```python
from build123d import *

# Parameters (mm, degrees)
SALIENTE_EXTRUIR4_DEPTH = 20
SALIENTE_EXTRUIR5_DEPTH = 30


with BuildPart() as part:
    # Croquis2 → Saliente-Extruir4 (new body)
    with BuildSketch(Plane(origin=(0, 0, 0), x_dir=(1, 0, 0), z_dir=(0, 1, 0))):
        Polygon((130, 20.207259422), (130, 24.997259422), (60, 24.997259422), (60, 44.997259422), (130, 44.997259422), (130, 49.792740578), (95, 70), (0, 70), (0, 0), (95, 0), align=None)
    extrude(amount=SALIENTE_EXTRUIR4_DEPTH)

    # Croquis4 → Saliente-Extruir5 (add)
    with BuildSketch(Plane.ZY):
        Polygon((0, 20), (0, 52.609160269), (-25, 52.609160269), (-16.339745962, 37.609160269), (-35, 37.609160269), (-35, 20), align=None)
    saliente_extruir5 = extrude(amount=-SALIENTE_EXTRUIR5_DEPTH)

    # Simetría1: Saliente-Extruir5 across plane
    add(saliente_extruir5.mirror(Plane(origin=(0, 0, -35), x_dir=(1, 0, 0), z_dir=(0, 0, -1))))


solid = part.part
```
Part model, mm, in its own coordinate system. A direction names the side the tool comes from. Round coordinates to 2 decimals unless told otherwise and drop trailing zeros. Loops run counter-clockwise (first coordinate to the right, second up) from the corner with the lowest first, then second, coordinate; pieces in that order, holes last. Notation, with made-up numbers: (-31.5, -2.5) -> (-8.5, -2.5) arc R4 ccw to (-8.5, 3.5) -> close; hole circle Ø8 at (7.5, -10.5). An arc over 180 degrees is marked (long way). Use one line per item in the form item = value. Start each with the question number.
Item 1: Band-saw the part on B-B (y = 41). List the corners of the cut face in (x, z), plus the area to 3 significant figures.
Item 2: Two-plate mould, pull along Y, no slides. Class faces 1 (the flat face through (14.79, 45.21, -20.73)), 2 (the flat face through (15, 52.609, -58)), 3 (the flat face through (130, 10, -23)): released by +Y, released by -Y, zero draft, split by the parting line, or undercut.
Item 3: Drill centre lines: line 1 along Y through (x, z) = (34, -60.5); line 2 along X through (y, z) = (27.5, -16); line 3 along Z through (x, y) = (10, 45). Where is each one in solid material? Low to high.
Item 4: Band-saw the part on A-A (x = 21.5). List the corners of the cut face in (y, z), plus the area to 3 significant figures.
Item 5: Drop flat-ended pins along their axis: pin 1 Ø8 at (x, y) = (100, 9) entering from -Z; pin 2 Ø10 at (y, z) = (30, -51.5) entering from +X. Give the stop position or say it passes through.
Item 6: Tool access for faces 4 (the flat face through (57, 20, -35)), 5 (the flat face through (95, 10, -24.997)), 6 (the flat face through (14.79, 45.21, -49.27)), 7 (the flat face through (112.745, 9.86, -59.755)): list every direction of +Z, -Z, +X, -X, +Y, -Y with a clear straight run to the whole face (end or side of a thin tool).
Item 7: Band-saw the part on D-D (y = 3). List the corners of the cut face in (x, z).
Item 8: Band-saw the part on C-C (x = 73). List the corners of the cut face in (y, z).
Data:
q1.outline = (0, -70) -> (30, -70) -> (30, -51.7) -> (0, -51.7) -> close; (0, -18.3) -> (30, -18.3) -> (30, 0) -> (0, 0) -> close
q1.area = 1,100 mm^2
q2.face_1 = undercut
q2.face_2 = released by +Y
q2.face_3 = zero draft
q3.line_1 = 0 to 20
q3.line_2 = 0 to 30
q3.line_3 = -70 to -49.39, -20.61 to 0
q4.outline = (0, -70) -> (52.61, -70) -> (52.61, -45) -> (37.61, -53.66) -> (37.61, -16.34) -> (52.61, -25) -> (52.61, 0) -> (0, 0) -> close
q4.area = 3,250 mm^2
q5.pin_1 = -69.42
q5.pin_2 = 30
q6.face_4 = +Z, -Z, +X, +Y
q6.face_5 = +X, +Y, -Y
q6.face_6 = +X, -X
q6.face_7 = -Z, +X, +Y, -Y
q7.outline = (0, -70) -> (95, -70) -> (130, -49.79) -> (130, -45) -> (60, -45) -> (60, -25) -> (130, -25) -> (130, -20.21) -> (95, 0) -> (0, 0) -> close
q8.outline = (0, -70) -> (20, -70) -> (20, -45) -> (0, -45) -> close; (0, -25) -> (20, -25) -> (20, 0) -> (0, 0) -> close
